Here's how the part is built. I have some questions about the finished solid (model axes, mm). Give positions to 0.01 mm unless a question says otherwise; leave off trailing zeros. Answer as CSV lines item,"result". Start each with the question number.
Item 1: Will this pin go through, and if not, where does the flat tip stop? P1, Ø3, axis at x = 294, y = -1.5, coming from the +Z side.
Item 2: I want a section at A-A on z = 6.25. Give the number of separate pieces and of enclosed holes in the cut face, plus the area to 3 significant figures.
Item 3: If I drill on line 1 along Y through (x, z) = (115, 15.25); line 2 along Z through (x, y) = (232, 0.5); line 3 along Y through (x, z) = (117.5, 11.5), over which ranges is the centre line in solid material (lowest first)? Write a range as from..to.
from build123d import *

# Parameters (mm, degrees)
SKETCH_W        = 800
SKETCH_H        = 20
PAD_DEPTH       = 17.5
SKETCH001_R     = 4.75
POCKET_DEPTH    = 8.5
SKETCH002_R     = 3
POCKET001_DEPTH = 17.501
CHAMFER_SIZE    = 1
SKETCH003_W     = 5
SKETCH003_H     = 5
POCKET002_DEPTH = 4


with BuildPart() as part:
    # Sketch → Pad (new body)
    with BuildSketch(Plane.XY):
        with Locations((385, 0)):
            Rectangle(SKETCH_W, SKETCH_H)
    extrude(amount=PAD_DEPTH)

    # Sketch001 (on Face6 of Pad) → Pocket (cut)
    with BuildSketch(Plane.XY.offset(17.5)):
        with Locations((-5, 0)):
            Circle(SKETCH001_R)
        with Locations((55, 0)):
            Circle(SKETCH001_R)
        with Locations((115, 0)):
            Circle(SKETCH001_R)
        with Locations((175, 0)):
            Circle(SKETCH001_R)
        with Locations((235, 0)):
            Circle(SKETCH001_R)
        with Locations((295, 0)):
            Circle(SKETCH001_R)
        with Locations((355, 0)):
            Circle(SKETCH001_R)
        with Locations((415, 0)):
            Circle(SKETCH001_R)
        with Locations((475, 0)):
            Circle(SKETCH001_R)
        with Locations((535, 0)):
            Circle(SKETCH001_R)
        with Locations((595, 0)):
            Circle(SKETCH001_R)
        with Locations((655, 0)):
            Circle(SKETCH001_R)
        with Locations((715, 0)):
            Circle(SKETCH001_R)
        with Locations((775, 0)):
            Circle(SKETCH001_R)
    extrude(amount=-POCKET_DEPTH, mode=Mode.SUBTRACT)

    # Sketch002 (on Face5 of Pocket) → Pocket001 (cut, through all)
    with BuildSketch(Plane.XY.offset(17.5)):
        with Locations((-5, 0)):
            Circle(SKETCH002_R)
        with Locations((55, 0)):
            Circle(SKETCH002_R)
        with Locations((115, 0)):
            Circle(SKETCH002_R)
        with Locations((175, 0)):
            Circle(SKETCH002_R)
        with Locations((235, 0)):
            Circle(SKETCH002_R)
        with Locations((295, 0)):
            Circle(SKETCH002_R)
        with Locations((355, 0)):
            Circle(SKETCH002_R)
        with Locations((415, 0)):
            Circle(SKETCH002_R)
        with Locations((475, 0)):
            Circle(SKETCH002_R)
        with Locations((535, 0)):
            Circle(SKETCH002_R)
        with Locations((595, 0)):
            Circle(SKETCH002_R)
        with Locations((655, 0)):
            Circle(SKETCH002_R)
        with Locations((715, 0)):
            Circle(SKETCH002_R)
        with Locations((775, 0)):
            Circle(SKETCH002_R)
    extrude(amount=-POCKET001_DEPTH, mode=Mode.SUBTRACT)

    # Chamfer
    chamfer_edges = [part.edges().sort_by_distance(p)[0] for p in [
        (785, 0, 17.5),
        (785, -10, 8.75),
        (785, 0, 0),
        (785, 10, 8.75),
        (385, 10, 17.5),
        (385, -10, 0),
        (385, 10, 0),
        (-15, 10, 8.75),
        (-15, 0, 17.5),
        (-15, -10, 8.75),
        (-15, 0, 0),
        (385, -10, 17.5),
    ]]
    chamfer(chamfer_edges, length=CHAMFER_SIZE)

    # Sketch003 → Pocket002 (cut)
    with BuildSketch(Plane.YZ):
        with Locations((0, 15)):
            Rectangle(SKETCH003_W, SKETCH003_H)
    extrude(amount=-POCKET002_DEPTH, mode=Mode.SUBTRACT)


solid = part.part
Result:
1,P1,"z = 9"
2,separate pieces,"1"
2,enclosed holes,"14"
2,area,"15,600 mm^2"
3,line 1,"-10..-4.75, 4.75..10"
3,line 2,"0..9"
3,line 3,"-10..-4.04, 4.04..10"
